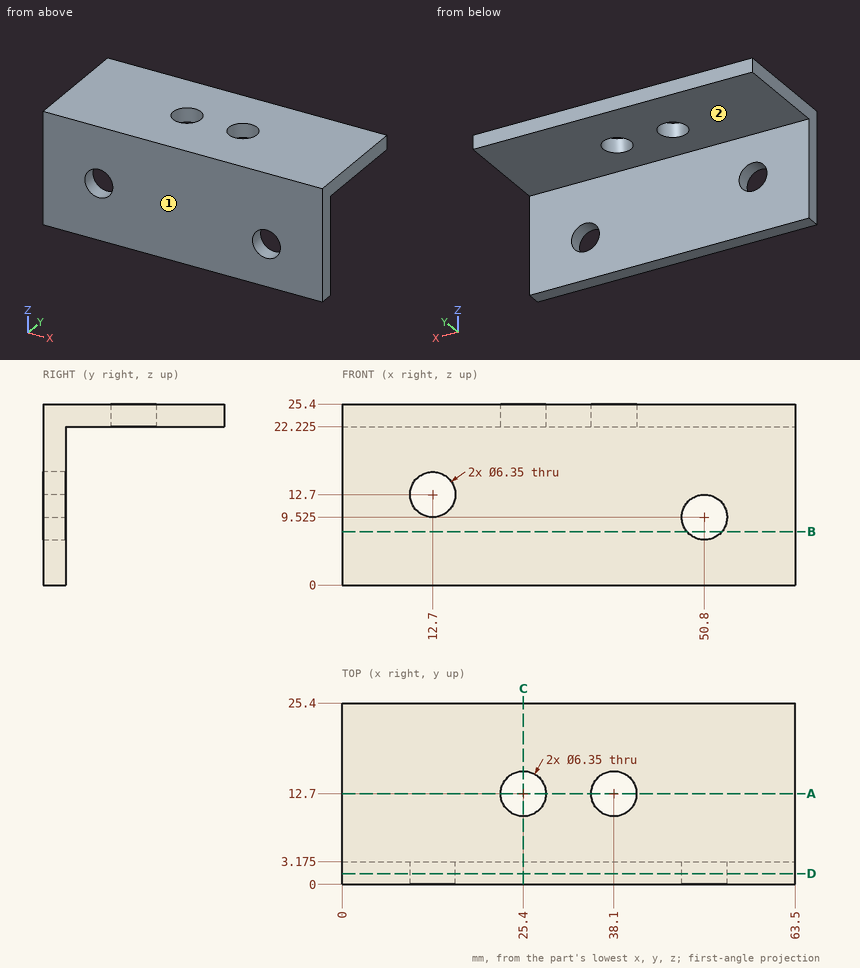
Source: three-view drawing plus pictorial views. Frame: mm from the lowest corner of the part. A direction names the side the tool comes from. Give positions to 0.01 mm unless a question says otherwise; leave off trailing zeros. Order: outer loops, then holes, each group sorted by start corner. A loop starts at its lowest first (then second) coordinate and runs counter-clockwise, first axis right, second up.
1. Section C-C on x = 25.4. Return the cut outline in (y, z) (3 decimals).
Derived:
outline: (0, 0) - (3.175, 0) - (3.175, 22.225) - (9.525, 22.225) - (9.525, 25.4) - (0, 25.4) - close; (15.875, 22.225) - (25.4, 22.225) - (25.4, 25.4) - (15.875, 25.4) - close
2. Section B-B on z = 7.5. Return the cut outline in (x, y) (3 decimals).
Derived:
outline: (0, 0) - (48.355, 0) - (48.355, 3.175) - (0, 3.175) - close; (53.245, 0) - (63.5, 0) - (63.5, 3.175) - (53.245, 3.175) - close
3. Section D-D on y = 1.5. Return the cut outline in (x, z) (3 decimals), and give its area (3 significant figures).
Derived:
outline: (0, 0) - (63.5, 0) - (63.5, 25.4) - (0, 25.4) - close; hole circle Ø6.35 at (12.7, 12.7); hole circle Ø6.35 at (50.8, 9.525)
area: 1,550 mm2
4. Section A-A on y = 12.7. Return the cut outline in (x, z) (3 decimals), and give its area (3 significant figures).
Derived:
outline: (0, 22.225) - (22.225, 22.225) - (22.225, 25.4) - (0, 25.4) - close; (28.575, 22.225) - (34.925, 22.225) - (34.925, 25.4) - (28.575, 25.4) - close; (41.275, 22.225) - (63.5, 22.225) - (63.5, 25.4) - (41.275, 25.4) - close
area: 161 mm2
5. Reachability of the marked faces 1 and 2 from +Z, -Z, +X, -X, +Y, -Y: full face, straight path, thin tool, end or side. Return the list, or none.
Derived:
face 1: +Z, -Z, +X, -X, -Y
face 2: -Z, +X, -X, +Y
6. Pin query (flat end, axial travel): pin 1 (5 mm diameter, centred on x = 50.8, z = 9.525, fed in from +Y); pin 2 (6 mm diameter, centred on x = 29, y = 21, fed in from -Z) (3 decimals); pin 3 (12 mm diameter, centred on x = 15, z = 4, fed in from +Y) (3 decimals). Return the tip coordinate at first contact, or that it passes through.
Derived:
pin 1: passes through
pin 2: stops at z = 22.225
pin 3: stops at y = 3.175
7. Material intervals for L1, parallel to Y at x = 25.4, z = 24.5 (3 decimals); L2, parallel to Z at x = 7, y = 16.25 (3 decimals); L3, parallel to Y at x = 49, z = 21.5 (3 decimals), sorted ascending.
Derived:
L1: y = 0 to 9.525, 15.875 to 25.4
L2: z = 22.225 to 25.4
L3: y = 0 to 3.175
